Read the model definition and answer for the solid it produces. Units are mm, in the model's axes. A direction names the side the tool comes from. Round coordinates to 2 decimals unless told otherwise and drop trailing zeros. Loops run counter-clockwise (first coordinate to the right, second up) from the corner with the lowest first, then second, coordinate; pieces in that order, holes last. Notation, with made-up numbers: M -37.5,-8.5 L -19.5,-8.5 A12 ccw -19.5,3.5 Z; hole C 32.25,31.25 d10. An arc over 180 degrees is marked long. Write each question's results on one line, items separated by ' | '.
```python
from build123d import *

# Parameters (mm, degrees)
SKETCH_W        = 100
SKETCH_H        = 62
PAD_DEPTH       = 4.45
SKETCH001_R     = 2
POCKET_DEPTH    = 4.45
SKETCH004_R     = 4.1
POCKET002_DEPTH = 5
SKETCH009_R     = 3.8
POCKET005_DEPTH = 5
SKETCH010_R     = 1.25
POCKET006_DEPTH = 5
SKETCH011_R     = 1.75
SKETCH011_R_2   = 2
POCKET007_DEPTH = 5
POCKET008_DEPTH = 5
SKETCH013_R     = 2
POCKET009_DEPTH = 5


with BuildPart() as part:
    # Sketch → Pad (new body)
    with BuildSketch(Plane.XY):
        with Locations((0, 1)):
            Rectangle(SKETCH_W, SKETCH_H)
    extrude(amount=PAD_DEPTH)

    # Sketch001 → Pocket (cut)
    with BuildSketch(Plane.XY.offset(4.45)):
        Circle(SKETCH001_R)
    extrude(amount=-POCKET_DEPTH, mode=Mode.SUBTRACT)

    # Sketch004 → Pocket002 (cut)
    with BuildSketch(Plane.XY.offset(4.45)):
        with Locations((-8, 0)):
            Circle(SKETCH004_R)
    extrude(amount=-POCKET002_DEPTH, mode=Mode.SUBTRACT)

    # Sketch009 → Pocket005 (cut)
    with BuildSketch(Plane.XY.offset(4.45)):
        with Locations((0, -22)):
            Circle(SKETCH009_R)
    extrude(amount=-POCKET005_DEPTH, mode=Mode.SUBTRACT)

    # Sketch010 → Pocket006 (cut)
    with BuildSketch(Plane.XZ.offset(30)):
        with Locations((0, 2.225)):
            Circle(SKETCH010_R)
    extrude(amount=-POCKET006_DEPTH, mode=Mode.SUBTRACT)

    # Sketch011 → Pocket007 (cut)
    with BuildSketch(Plane.XY.offset(4.45)):
        with Locations((-16, 0)):
            Circle(SKETCH011_R)
        with Locations((-32, 0)):
            Circle(SKETCH011_R_2)
    extrude(amount=-POCKET007_DEPTH, mode=Mode.SUBTRACT)

    # Sketch012 → Pocket008 (cut)
    with BuildSketch(Plane.XY.offset(4.45)):
        with BuildLine():
            ThreePointArc((14, 20), (12, 22), (10, 20))
            Line((10, 20), (10, 10))
            ThreePointArc((10, 10), (12, 8), (14, 10))
            Line((14, 20), (14, 10))
        make_face()
        with BuildLine():
            ThreePointArc((-10, 20), (-11.999997, 22.000006), (-14, 20.000006))
            Line((-14, 20.000006), (-14, 10.00001))
            ThreePointArc((-14, 10.00001), (-12.000005, 8.000011), (-10, 10))
            Line((-10, 20), (-10, 10))
        make_face()
    extrude(amount=-POCKET008_DEPTH, mode=Mode.SUBTRACT)

    # Sketch013 → Pocket009 (cut)
    with BuildSketch(Plane.XY.offset(4.45)):
        with Locations((44, 27.45)):
            Circle(SKETCH013_R)
        with Locations((-44, 27.45)):
            Circle(SKETCH013_R)
        with Locations((0, 27.45)):
            Circle(SKETCH013_R)
    extrude(amount=-POCKET009_DEPTH, mode=Mode.SUBTRACT)


solid = part.part
```
1. Find the intervals of material crossed by L1, parallel to Y at x = 0, z = 2.05; L2, parallel to X at y = 1.5, z = 3.85; L3, parallel to X at y = 19, z = 1.45, in increasing order.
Completed:
L1: y = -18.2 to -2, 2 to 25.45, 29.45 to 32 | L2: x = -50 to -33.32, -30.68 to -16.9, -15.1 to -11.82, -4.18 to -1.32, 1.32 to 50 | L3: x = -50 to -14, -10 to 10, 14 to 50
2. Find section C-C, the plane x = 44. Give the vertices of the cut face in (y, z).
Completed:
outline: M -30,0 L 25.45,0 L 25.45,4.45 L -30,4.45 Z; M 29.45,0 L 32,0 L 32,4.45 L 29.45,4.45 Z
3. Find section B-B, the plane x = 12. Give the vertices of the cut face in (y, z), then the cut area to 3 significant figures.
Completed:
outline: M -30,0 L 8,0 L 8,4.45 L -30,4.45 Z; M 22,0 L 32,0 L 32,4.45 L 22,4.45 Z | area: 214 mm2
4. Which of the six approach directions +Z, -Z, +X, -X, +Y, -Y give full straight-line access (tool end or side, diameter ignored) to faces 4 (the face through (-0.271, -27.822, 1.005)), 5 (the face through (-50, 1, 2)), 6 (the face through (-10, 15, 2))?
Completed:
face 4: -Y | face 5: +Z, -Z, -X, +Y, -Y | face 6: +Z, -Z
5. Find section A-A, the plane x = 0. Give the vertices of the cut face in (y, z) (3 decimals).
Completed:
outline: M -30,0 L -25.8,0 L -25.8,0.975 L -30,0.975 Z; M -30,3.475 L -25.8,3.475 L -25.8,4.45 L -30,4.45 Z; M -18.2,0 L -2,0 L -2,4.45 L -18.2,4.45 Z; M 2,0 L 25.45,0 L 25.45,4.45 L 2,4.45 Z; M 29.45,0 L 32,0 L 32,4.45 L 29.45,4.45 Z
6. Determine the mould class of faces 1 (the face through (-1, -5, 4.45)), 2 (the face through (-1, -30, 4)), 3 (the face through (12, 22, 2)) for opening direction Y: released by +Y, released by -Y, zero draft, split by the parting line, or undercut.
Completed:
face 1: zero draft | face 2: released by -Y | face 3: undercut
